Model file for the job. Use its own axes, mm. Coordinates: 2 decimals unless noted, no trailing zeros. Order: outer loops, then holes, each group sorted by start corner. A loop starts at its lowest first (then second) coordinate and runs counter-clockwise, first axis right, second up. Notation, with made-up numbers: M 5,0 L 37,0 A24 cw 37,21 Z; hole C -7.75,24.25 d3. An arc over 180 degrees is marked long. Return JSON: item names as keys, results as strings.
```python
from build123d import *

# Parameters (mm, degrees)
F2_R = 3
F3_R = 0.5


with BuildPart() as f1:
    # F0 (on Front) → F1 (revolve)
    with BuildSketch(Plane.XZ):
        Polygon((0, 1), (0, 0), (15.8, 0), (6.8, 18.462429), (3.8, 17), align=None)
    revolve(axis=Axis((0, 0, 0.5), (0, 0, -1)))

    # F2
    f2_edges = [f1.edges().sort_by_distance(p)[0] for p in [
        (-3.8, 0, 17),
        (1.9, 0, 9),
    ]]
    fillet(f2_edges, radius=F2_R)

    # F3
    f3_edges = [f1.edges().sort_by_distance(p)[0] for p in [
        (-6.8, 0, 18.462429),
    ]]
    fillet(f3_edges, radius=F3_R)


solid = f1.part
```
Item 1: Drop flat-ended pins along their axis: pin 1 Ø6 at (x, z) = (-3.5, 5) entering from +Y; pin 2 Ø3 at (x, y) = (-6, 12) entering from +Z; pin 3 Ø1 at (x, z) = (-9, 9.5) entering from -Y. Give the stop position or say it passes through.
Check result:
{"pin 1": "stops at y = 14.53", "pin 2": "stops at z = 7.97", "pin 3": "stops at y = -7.36"}
Item 2: Pull direction Y, two halves, no side cores. Call faces 1 (the conical face through (-1.36, 1.04, 8.21)), 2 (the flat face through (0, 0, 0)), 3 (the conical face through (-2, 9.2, 13.1)): +Y half, -Y half, draft (parallel to the pull), parting line (faces both ways), or undercut.
Check result:
{"face 1": "undercut", "face 2": "draft", "face 3": "parting line"}
Item 3: Saw through at B-B (z = 12). Write the cut outline in (x, y) (1 decimal), and give its area (3 significant figures).
Check result:
{"outline": "C 0,0 d19.9; hole C 0,0 d5.2", "area": "290 mm2"}
Item 4: Saw through at A-A (z = 3.75). Write the cut outline in (x, y).
Check result:
{"outline": "C 0,0 d27.94; hole C 0,0 d1.31"}
Item 5: Wall check: line 1 (X direction, y = 2, z = 13.75); line 2 (Y direction, x = -1, z = 17.5); line 3 (X direction, y = -1, z = 8.25). Give the ranges that are in metal, low to high.
Check result:
{"line 1": "x = -8.87 to -2.27, 2.27 to 8.87", "line 2": "y = -7.2 to -4.75, 4.75 to 7.2", "line 3": "x = -11.74 to -1.4, 1.4 to 11.74"}
